Input: part model. Units: mm. Frame: model coordinates. Face numbers are marked on the shaded views. A direction names the side the tool comes from. Coordinates: 2 decimals unless noted, no trailing zeros. Order: outer loops, then holes, each group sorted by start corner. A loop starts at its lowest first (then second) coordinate and runs counter-clockwise, first axis right, second up. Notation, with made-up numbers: M 76.5,30.5 L 107.5,30.5 A21 cw 107.5,59.5 Z; hole C 24,-2 d8. An arc over 180 degrees is marked long. One line per item, written item: value.
```python
from build123d import *

# Parameters (mm, degrees)
F2_R     = 0.49999
F3_SIZE2 = 0.25
F3_SIZE  = 0.25


# Not quite as in the source:
# - a fillet or chamfer is up to 0.001 mm smaller than in the source, because OpenCascade refuses the exact size


with BuildPart() as f1:
    # F0 (on Front) → F1 (revolve)
    with BuildSketch(Plane.XZ):
        Polygon((0, 8), (0, 0), (0.8, 0), (0.8, 2), (1.5, 2), (1.5, 7), (2, 7), (2, 8), align=None)
    revolve(axis=Axis((0, 0, 4), (0, 0, 1)))

    # F2 (radius 0.5 in the source; OpenCascade refuses exactly that, so slightly less here)
    f2_edges = [f1.edges().sort_by_distance(p)[0] for p in [
        (-2, 0, 7),
        (-2, 0, 8),
        (2, 0, 7.5),
        (-1.5, 0, 2),
    ]]
    fillet(f2_edges, radius=F2_R)

    # F3
    f3_edges = [f1.edges().sort_by_distance(p)[0] for p in [
        (-0.8, 0, 0),
    ]]
    chamfer(f3_edges, length=F3_SIZE, length2=F3_SIZE2)


solid = f1.part
```
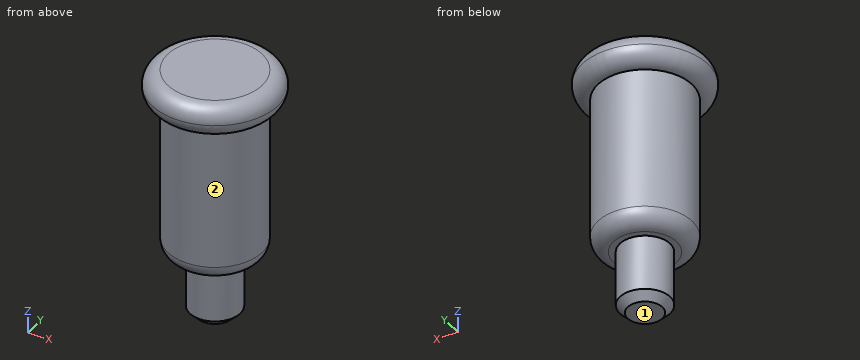
(1) Access query for the marked faces 1 and 2. Directions: +Z, -Z, +X, -X, +Y, -Y. A direction counts if a zero-diameter tool reaches every point of the face in a straight line with its end or side. Return the directions, or none.
Data:
face 1: -Z, +X, -X, +Y, -Y
face 2: -Z
(2) Cut plane C-C on z = 1.25. Output: boundary loops of the cut face in (x, y).
Data:
outline: C 0,0 d1.6
(3) Ray query, line 1 (Z direction, x = -0.5, y = -0.9); line 2 (Y direction, x = 0.05, z = 0.5); line 3 (Y direction, x = -0.05, z = 7.25). Return the intervals inside material, ascending. Write a range as from..to.
Data:
line 1: z = 2..8
line 2: y = -0.8..0.8
line 3: y = -1.93..1.93
(4) First-contact query: pin 1 (1 mm diameter, centred on y = -1, z = 5.5, fed in from +X). Flat tip, straight axial feed; report the tip coordinate or a pass-through.
Data:
pin 1: stops at x = 1.41
(5) Cut plane D-D on z = 5.5. Output: boundary loops of the cut face in (x, y), plus the area to 3 significant figures.
Data:
outline: C 0,0 d3
area: 7.07 mm2
